from build123d import *

# Parameters (mm, degrees)
SKETCH1_W           = 51.53
SKETCH1_H           = 30
BOSS_EXTRUDE1_DEPTH = 5
CUT_EXTRUDE1_DEPTH  = 5
SKETCH4_R           = 1.5
CUT_EXTRUDE3_DEPTH  = 5


with BuildPart() as part:
    # Sketch1 → Boss-Extrude1 (new body)
    with BuildSketch(Plane.XY):
        with Locations((2.765, -5)):
            Rectangle(SKETCH1_W, SKETCH1_H)
    extrude(amount=BOSS_EXTRUDE1_DEPTH)

    # Sketch2 → Cut-Extrude1 (cut)
    with BuildSketch(Plane.XY.offset(5)):
        Polygon((13.53, -1.9), (20.865904873, -1.9), (20.865904873, -3.4), (24.265904873, -3.4), (24.265904873, -1.9), (28.53, -1.9), (28.53, 2.5), (24.265904873, 2.5), (24.265904873, 4), (20.865904873, 4), (20.865904873, 2.5), (13.53, 2.5), align=None)
        Polygon((4.13, -5), (4.13, -11.6), (2.63, -11.6), (2.63, -15), (4.13, -15), (4.13, -20), (8.53, -20), (8.53, -15), (10.03, -15), (10.03, -11.6), (8.53, -11.6), (8.53, -5), align=None)
    extrude(amount=-CUT_EXTRUDE1_DEPTH, mode=Mode.SUBTRACT)

    # Sketch4 → Cut-Extrude3 (cut)
    with BuildSketch(Plane.XY.offset(5)):
        with Locations((-13.899616309, -4.903624059)):
            Circle(SKETCH4_R)
    extrude(amount=-CUT_EXTRUDE3_DEPTH, mode=Mode.SUBTRACT)


solid = part.part
Input: part model. Units: mm. Frame: model coordinates. A direction names the side the tool comes from. Give positions to 0.01 mm unless a question says otherwise; leave off trailing zeros. Loops run counter-clockwise (first coordinate to the right, second up) from the corner with the lowest first, then second, coordinate; pieces in that order, holes last. Notation, with made-up numbers: (-27, 65) - (-5, 65) arc R24 ccw to (-5, 84) - close; hole circle Ø2 at (24, 42.25). An arc over 180 degrees is marked (long way). Use CSV: the item, a comma, the result in double quotes. Start each with the question number.
Item 1: Mould query, pull axis X, two halves, no side actions, for faces 1 (the flat face through (13.53, 0, 3)), 2 (the flat face through (4.13, -8, 3)), 3 (the flat face through (17, 2.5, 3)). Classes: pulls with the +X half, pulls with the -X half, needs draft (parallel to the pull), parting line crosses it, or undercut.
Item 2: Section A-A on y = -17. Return loops of the section in (x, z), then the cut area to 3 significant figures.
Item 3: Reachability of faces 4 (the flat face through (6, -5, 3)), 5 (the flat face through (24.266, 3, 3)), 6 (the flat face through (26, 2.5, 3)) from +Z, -Z, +X, -X, +Y, -Y: full face, straight path, thin tool, end or side. Return the list, or none.
Item 4: Section D-D on y = -0.75. Return loops of the section in (x, z).
Item 5: Contact query for a flat-ended pin moving along its axis: P1, Ø2, axis at x = 7, z = 1.5, coming from the -Y side. Output: stop coordinate, or through.
Item 6: Line query: line 1 (X direction, y = -9.75, z = 2.95); line 2 (X direction, y = -2.5, z = 2.4); line 3 (Y direction, x = 22, z = 3). Output: solid intervals per line, ascending.
Item 7: Section B-B on x = 15. Return loops of the section in (y, z), then the cut area to 3 significant figures.
Ans:
1,face 1,"pulls with the +X half"
1,face 2,"undercut"
1,face 3,"needs draft"
2,outline,"(-23, 0) - (4.13, 0) - (4.13, 5) - (-23, 5) - close; (8.53, 0) - (28.53, 0) - (28.53, 5) - (8.53, 5) - close"
2,area,"236 mm2"
3,face 4,"+Z, -Z, -Y"
3,face 5,"+Z, -Z"
3,face 6,"+Z, -Z, +X"
4,outline,"(-23, 0) - (13.53, 0) - (13.53, 5) - (-23, 5) - close"
5,P1,"stops at y = -5"
6,line 1,"x = -23 to 4.13, 8.53 to 28.53"
6,line 2,"x = -23 to 20.87, 24.27 to 28.53"
6,line 3,"y = -20 to -3.4, 4 to 10"
7,outline,"(-20, 0) - (-1.9, 0) - (-1.9, 5) - (-20, 5) - close; (2.5, 0) - (10, 0) - (10, 5) - (2.5, 5) - close"
7,area,"128 mm2"
